CAD build for the part. Positions are in the model's coordinates, mm. Face numbers are marked on the shaded views. A direction names the side the tool comes from. Coordinates: 2 decimals unless noted, no trailing zeros. Order: outer loops, then holes, each group sorted by start corner. A loop starts at its lowest first (then second) coordinate and runs counter-clockwise, first axis right, second up.
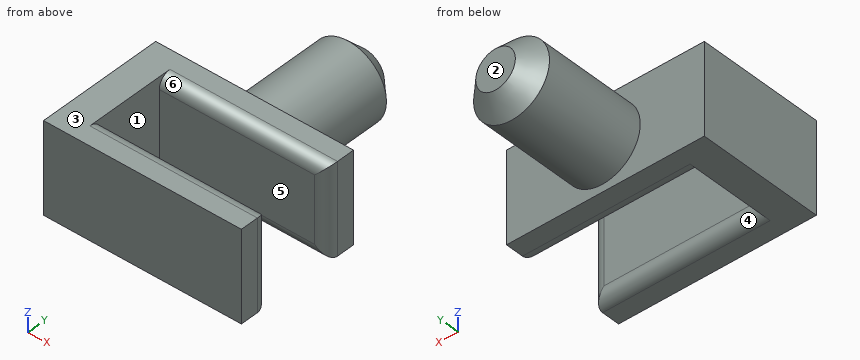
from build123d import *

# Parameters (mm, degrees)
F1_DEPTH = 7.5
F2_R     = 6.272579
F3_DEPTH = 20
F4_SIZE  = 3
F5_R     = 2


with BuildPart() as f1:
    # F0 (on Top) → F1 (new body, symmetric)
    with BuildSketch(Plane.XY):
        Polygon((15.831904, -5), (15.831904, 0), (-16.857163, 0), (-16.857163, -21), (15.831904, -21), (15.831904, -16), (-11.857163, -16), (-11.857163, -5), align=None)
    extrude(amount=F1_DEPTH, both=True)

    # F2 (on Front) → F3 (join)
    with BuildSketch(Plane.XZ):
        Circle(F2_R)
    extrude(amount=-F3_DEPTH)

    # F4
    f4_edges = [f1.edges().sort_by_distance(p)[0] for p in [
        (-6.272579, 20, 0),
    ]]
    chamfer(f4_edges, length=F4_SIZE)

    # F5
    f5_edges = [f1.edges().sort_by_distance(p)[0] for p in [
        (1.98737, -5, -7.5),
        (1.98737, -16, -7.5),
        (15.831904, -16, 0),
        (15.831904, -5, 0),
        (1.98737, -5, 7.5),
        (1.98737, -16, 7.5),
    ]]
    fillet(f5_edges, radius=F5_R)


solid = f1.part
1) Pin check, flat tips, straight feed: P1, Ø1, axis at x = -8, z = 3.5, coming from the +Y side; P2, Ø1, axis at y = 11, z = -5.5, coming from the +X side; P3, Ø10, axis at x = 8.5, y = 8, coming from the +Z side. Stop position of each tip, or through.
2) Slice it at C-C (x = 12.5). List the corners of the cut face in (y, z).
3) Slice it at D-D (y = -13). List the corners of the cut face in (x, z), plus the area to 3 significant figures.
4) Drill centre lines: probe 1 along Y at (x, z) = (-1, 1.25); probe 2 along Y at (x, z) = (14, 0.5); probe 3 along Y at (x, z) = (-14.5, -2). Where is each one in solid material? Low to high.
5) Slice it at B-B (z = 0). List the corners of the cut face in (x, y), plus the area to 3 significant figures.
6) Slice it at A-A (x = 0). List the corners of the cut face in (y, z).
7) Two-plate mould, pull along Y, no slides. Class the marked faces 1, 2 and 3: released by +Y, released by -Y, zero draft, split by the parting line, or undercut.
8) Which spindle directions (+Z, -Z, +X, -X, +Y, -Y) get a long thin tool onto all of the face, cutting with end or side? Do the marked faces 4, 5 and 6. Say none if no direction does.
Worked out:
1. P1: stops at y = 0
1. P2: stops at x = 3.79
1. P3: stops at z = 5.21
2. outline: (-21, -7.5) - (-18, -7.5) arc R2 ccw to (-16, -5.5) - (-16, 5.5) arc R2 ccw to (-18, 7.5) - (-21, 7.5) - close; (-5, -5.5) arc R2 ccw to (-3, -7.5) - (0, -7.5) - (0, 7.5) - (-3, 7.5) arc R2 ccw to (-5, 5.5) - close
3. outline: (-16.86, -7.5) - (-11.86, -7.5) - (-11.86, 7.5) - (-16.86, 7.5) - close
3. area: 75.0 mm2
4. probe 1: y = -21 to -16, -5 to 20
4. probe 2: y = -21 to -16.01, -4.99 to 0
4. probe 3: y = -21 to 0
5. outline: (-16.86, -21) - (15.83, -21) - (15.83, -18) arc R2 ccw to (13.83, -16) - (-11.86, -16) - (-11.86, -5) - (13.83, -5) arc R2 ccw to (15.83, -3) - (15.83, 0) - (6.27, 0) - (6.27, 17) - (3.27, 20) - (-3.27, 20) - (-6.27, 17) - (-6.27, 0) - (-16.86, 0) - close
5. area: 622 mm2
6. outline: (-21, -7.5) - (-18, -7.5) arc R2 ccw to (-16, -5.5) - (-16, 5.5) arc R2 ccw to (-18, 7.5) - (-21, 7.5) - close; (-5, -5.5) arc R2 ccw to (-3, -7.5) - (0, -7.5) - (0, -6.27) - (17, -6.27) - (20, -3.27) - (20, 3.27) - (17, 6.27) - (0, 6.27) - (0, 7.5) - (-3, 7.5) arc R2 ccw to (-5, 5.5) - close
7. face 1: undercut
7. face 2: released by +Y
7. face 3: zero draft
8. face 4: -Z, +X
8. face 5: +Z, -Z, +X
8. face 6: +Z, +X
